Geometry: final body of the model. Coordinates: model frame, mm. Coordinates: 2 decimals unless noted, no trailing zeros. Write each loop counter-clockwise with the first axis right and the second up, starting at its lowest first coordinate (ties: lowest second). Pieces come first, ordered by that corner, then holes.
Autodesk Inventor part; units mm, degrees
ref_plane "YZ Plane" through (0, 0, 0) normal (1, 0, 0) x (0, 1, 0)
ref_plane "XZ Plane" through (0, 0, 0) normal (0, 1, 0) x (-1, 0, 0)
ref_plane "XY Plane" through (0, 0, 0) normal (0, 0, 1) x (1, 0, 0)
sketch "Sketch1" plane through (0, 0, 0) normal (1, 0, 0) x (0, 1, 0)
  line L0 (0, 0) -> (30, 0)
  line L1 (30, 0) -> (30, -20)
  line L2 (30, -20) -> (0, -20)
  line L3 (0, -20) -> (0, 0)
  dimension "d0" = 20
  dimension "d1" = 30
extrude "Extrusion1" add sketch "Sketch1" against normal blind 300
sketch "Sketch3" plane through (0, 0, 0) normal (1, 0, 0) x (0, 0, -1)
  line L0 (0, 0) -> (0, 30)
  line L1 (0, 0) -> (0, 30)
  line L2 (0, 30) -> (-30, 30)
  line L3 (-30, 30) -> (0, 0)
  dimension "d4" = 30
  dimension "d5" = 45
extrude "Extrusion2" add sketch "Sketch3" along normal blind 300 from surface at -300
sketch "Sketch4" plane through (0, 0, 0) normal (1, 0, 0) x (0, 0, -1)
  line L0 (0, 0) -> (20, 0)
  line L1 (20, 0) -> (20, 30)
  line L2 (20, 30) -> (0, 30)
  line L3 (0, 30) -> (0, 0)
extrude "Extrusion3" cut sketch "Sketch4" against normal through all
properties part number "cale_monnayeur"
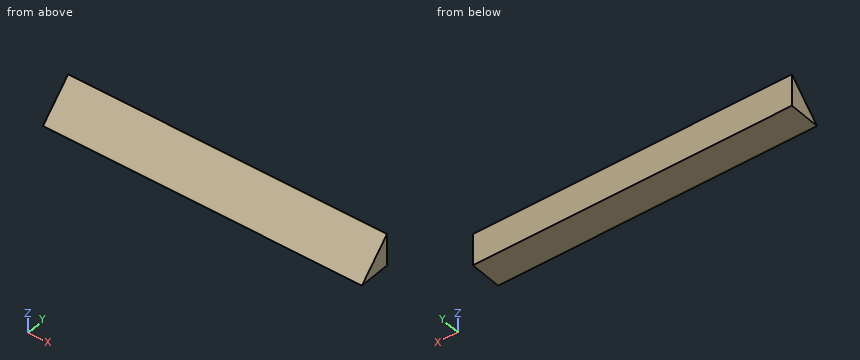
Item 1: Section B-B, the plane y = 21. Output: boundary loops of the cut face in (x, z).
Derived:
outline: (-300, 0) - (0, 0) - (0, 21) - (-300, 21) - close
Item 2: Material intervals for probe 1 along Y at (x, z) = (-197, 10.5); probe 2 along Z at (x, y) = (-258, 28); probe 3 along Y at (x, z) = (-37, 9.5), sorted ascending.
Derived:
probe 1: y = 10.5 to 30
probe 2: z = 0 to 28
probe 3: y = 9.5 to 30
Item 3: Section C-C, the plane x = -32. Output: boundary loops of the cut face in (y, z), plus the area to 3 significant figures.
Derived:
outline: (0, 0) - (30, 0) - (30, 30) - close
area: 450 mm2
Item 4: Section A-A, the plane z = 2.5. Output: boundary loops of the cut face in (x, y), plus the area to 3 significant figures.
Derived:
outline: (-300, 2.5) - (0, 2.5) - (0, 30) - (-300, 30) - close
area: 8,250 mm2
